Check sheet for the drawn part. Datum: minimum x, y, z corner. Units: mm. Give positions to 0.01 mm unless a question says otherwise; leave off trailing zeros. Order: outer loops, then holes, each group sorted by start corner. A loop starts at its lowest first (then second) coordinate and runs counter-clockwise, first axis right, second up. Notation, with made-up numbers: (-25.5, -5) -> (-13.5, -5) arc R29 ccw to (-13.5, 20) -> close; hole circle Ø11 at (-25, -19). An arc over 180 degrees is marked (long way). Answer in a Markdown table with one row per item. Add a question column.
(1) Cross-section at B-B (x = 21). Record the cut outline in (y, z) (3 decimals), then the cut area to 3 significant figures.
(2) Thickness scan on L1, parallel to X at y = 1.4, z = 25; L2, parallel to Z at x = 5, y = 1.95; L3, parallel to X at y = 2.95, z = 83.5. Record the ranges inside material, lowest first. Write a range as [from, to].
(3) Go/stop test with a flat-tipped pin: pin 1 (3.5 mm diameter, centred on x = 5, z = 25, fed in from -Y). Record where the tip stops, or that it passes through.
(4) Cross-section at D-D (z = 90.5). Record the cut outline in (x, y) (3 decimals), then the cut area to 3 significant figures.
(5) Cross-section at A-A (y = 2.1). State how many separate pieces and enclosed holes the cut face has, then the cut area to 3 significant figures.
(6) Cross-section at C-C (z = 25). Record the cut outline in (x, y) (3 decimals).
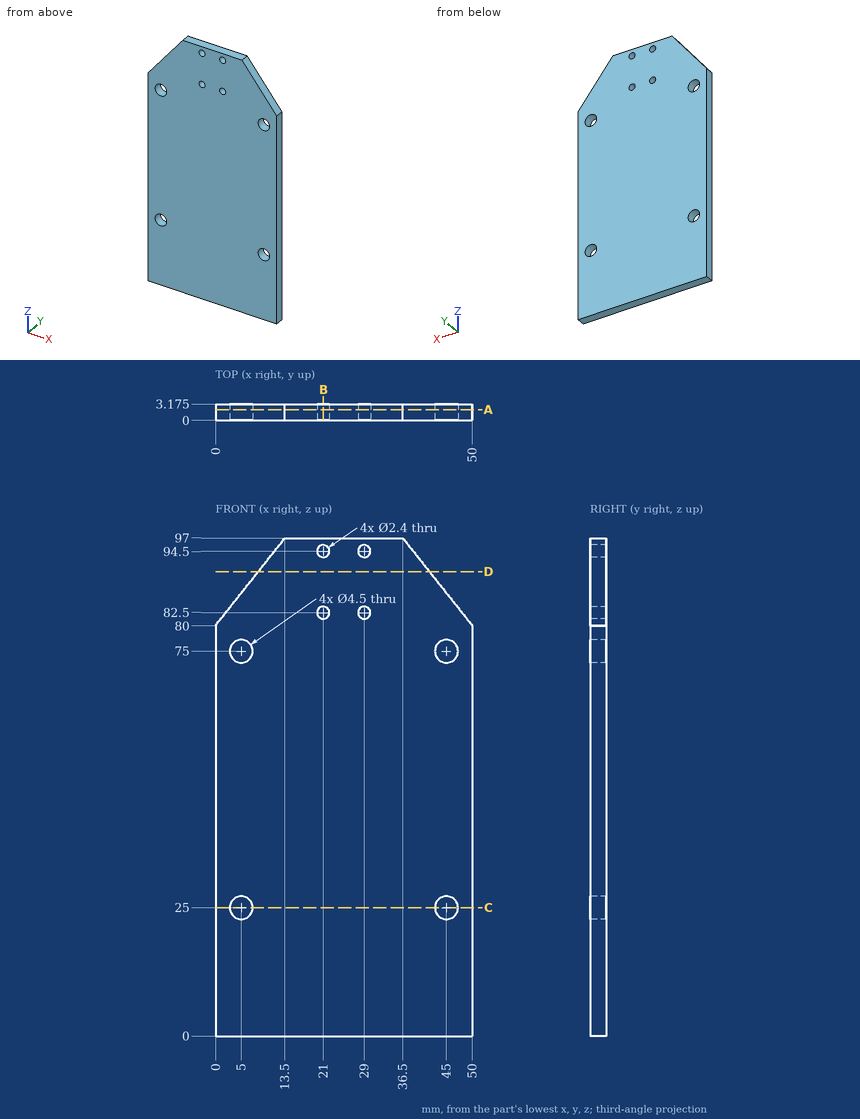
Answer below:
| question | item | result |
|---|---|---|
| 1 | outline | (0, 0) -> (3.175, 0) -> (3.175, 81.3) -> (0, 81.3) -> close; (0, 83.7) -> (3.175, 83.7) -> (3.175, 93.3) -> (0, 93.3) -> close; (0, 95.7) -> (3.175, 95.7) -> (3.175, 97) -> (0, 97) -> close |
| 1 | area | 293 mm² |
| 2 | L1 | x = [0, 2.75], [7.25, 42.75], [47.25, 50] |
| 2 | L2 | z = [0, 22.75], [27.25, 72.75], [77.25, 86.3] |
| 2 | L3 | x = [2.78, 20.34], [21.66, 28.34], [29.66, 47.22] |
| 3 | pin 1 | passes through |
| 4 | outline | (8.338, 0) -> (41.662, 0) -> (41.662, 3.175) -> (8.338, 3.175) -> close |
| 4 | area | 106 mm² |
| 5 | separate pieces | 1 |
| 5 | enclosed holes | 8 |
| 5 | area | 4,540 mm² |
| 6 | outline | (0, 0) -> (2.75, 0) -> (2.75, 3.175) -> (0, 3.175) -> close; (7.25, 0) -> (42.75, 0) -> (42.75, 3.175) -> (7.25, 3.175) -> close; (47.25, 0) -> (50, 0) -> (50, 3.175) -> (47.25, 3.175) -> close |
